Autodesk Inventor part; units mm, degrees
ref_plane "YZ Plane" through (0, 0, 0) normal (1, 0, 0) x (0, 1, 0)
ref_plane "XZ Plane" through (0, 0, 0) normal (0, 1, 0) x (-1, 0, 0)
ref_plane "XY Plane" through (0, 0, 0) normal (0, 0, 1) x (1, 0, 0)
sketch "Sketch1" plane through (0, 0, 0) normal (1, 0, 0) x (0, 1, 0)
  line L0 (9.8481, 428.814) -> (120.1519, 448.2635)
  line L1 (131.7365, 440.1519) -> (154.2135, 312.6787)
  line L2 (0, 78.3368) -> (0, 427.0775)
  line L3 (0, 417.0775) -> (0, 78.3368)
  line L4 (503.1119, 189.3047) -> (590.8645, 150.2346)
  line L5 (595.9326, 137.0318) -> (559.5861, 55.3964)
  line L6 (494.9423, 192.942) -> (494.9423, 192.942)
  line L7 (442.0149, 172.9748) -> (165.6696, 297.928)
  arc A0 (442.0149, 172.9748) -> (490.9347, 186.0198) centre (458.495, 209.4221) ccw
  arc A1 (154.2135, 312.6787) -> (165.6696, 297.928) centre (173.9096, 316.1516) ccw
  arc A2 (131.7365, 440.1519) -> (120.1519, 448.2635) centre (121.8884, 438.4154) ccw
  line L8 (9.8481, 428.814) -> (0, 417.0775)
  arc A3 (595.9326, 137.0318) -> (590.8645, 150.2346) centre (586.7972, 141.0991) ccw
  arc A4 (503.1119, 189.3047) -> (490.9347, 186.0198) centre (499.0446, 180.1692) ccw
  line L9 (9.651, 68.3429) -> (550.1017, 49.4699)
  arc A5 (550.1017, 49.4699) -> (559.5861, 55.3964) centre (550.4507, 59.4638) ccw
  arc A6 (0, 78.3368) -> (9.651, 68.3429) centre (10, 78.3368) ccw
  point P0 (0, 0)
  point P1 (0, 0)
  point P2 (130, 450)
  point P3 (156.0472, 302.2788)
  point P4 (0, 0)
  point P5 (534.922, 0)
  point P6 (600, 146.1672)
  point P7 (478.4622, 156.4947)
  point P8 (0, 427.0775)
  point P9 (537.6655, 6.1619)
  point P10 (0, 417.0775)
  dimension "d0" = 130
  dimension "d1" = 404.922
  dimension "d3" = 150
  dimension "d5" = 115
  dimension "d7" = 10
  dimension "d9" = 40
  dimension "d10" = 40
  dimension "d11" = 20
  dimension "d12" = 10
  dimension "d13" = 10
  dimension "d14" = 10
  dimension "d21" = 10
extrude "Extrusion1" add sketch "Sketch1" along normal blind 15
sketch "Sketch2" plane through (0, 0, 0) normal (-1, 0, 0) x (0, 0, 1)
  point P0 (0, 0)
sketch "Sketch3" plane through (0, 0, 0) normal (-1, 0, 0) x (0, 0, 1)
  line L0 (171.0338, 494.9772) -> (173.8576, 488.6347)
  line L1 (166.9664, 504.1126) -> (130.324, 487.7983)
  line L2 (130.324, 487.7983) -> (274.7158, 163.4898)
  line L3 (274.7158, 163.4898) -> (219.9031, 139.0856)
  line L4 (219.9031, 139.0856) -> (223.9704, 129.9501)
  line L5 (223.9704, 129.9501) -> (278.7831, 154.3544)
  line L6 (278.7831, 154.3544) -> (288.9516, 131.5158)
  line L7 (288.9516, 131.5158) -> (298.087, 135.5831)
  line L8 (298.087, 135.5831) -> (143.5268, 482.7303)
  line L9 (143.5268, 482.7303) -> (171.0338, 494.9772)
  line L10 (173.8576, 488.6347) -> (182.9931, 492.702)
  line L11 (182.9931, 492.702) -> (141.0991, 586.7972)
  line L12 (141.0991, 586.7972) -> (131.9637, 582.7298)
  line L13 (301.7603, 135.8301) -> (426.8309, 113.7768)
  line L14 (426.8309, 113.7768) -> (407.5559, 4.4631)
  line L15 (407.5559, 4.4631) -> (417.404, 2.7267)
  line L16 (417.404, 2.7267) -> (438.4154, 121.8884)
  line L17 (438.4154, 121.8884) -> (303.4968, 145.6782)
  line L18 (303.4968, 145.6782) -> (301.7603, 135.8301)
  line L19 (428.814, 9.8481) -> (417.0775, 0)
  line L20 (417.0775, 0) -> (78.3368, 0)
  line L21 (55.3964, 559.5861) -> (137.0318, 595.9326)
  arc A0 (150.2346, 590.8645) -> (137.0318, 595.9326) centre (141.0991, 586.7972) ccw
  line L22 (150.2346, 590.8645) -> (189.3047, 503.1119)
  arc A1 (186.0198, 490.9347) -> (189.3047, 503.1119) centre (180.1692, 499.0446) ccw
  arc A2 (186.0198, 490.9347) -> (172.9748, 442.0149) centre (209.4221, 458.495) ccw
  line L23 (172.9748, 442.0149) -> (297.928, 165.6696)
  arc A3 (297.928, 165.6696) -> (312.6787, 154.2135) centre (316.1516, 173.9096) ccw
  line L24 (312.6787, 154.2135) -> (440.1519, 131.7365)
  arc A4 (448.2635, 120.1519) -> (440.1519, 131.7365) centre (438.4154, 121.8884) ccw
  line L25 (448.2635, 120.1519) -> (428.814, 9.8481)
  line L26 (171.0338, 494.9772) -> (173.8576, 488.6347)
  line L27 (166.9664, 504.1126) -> (130.324, 487.7983)
  line L28 (130.324, 487.7983) -> (274.7158, 163.4898)
  line L29 (274.7158, 163.4898) -> (219.9031, 139.0856)
  line L30 (219.9031, 139.0856) -> (223.9704, 129.9501)
  line L31 (223.9704, 129.9501) -> (278.7831, 154.3544)
  line L32 (278.7831, 154.3544) -> (288.9516, 131.5158)
  line L33 (288.9516, 131.5158) -> (298.087, 135.5831)
  line L34 (298.087, 135.5831) -> (143.5268, 482.7303)
  line L35 (143.5268, 482.7303) -> (171.0338, 494.9772)
  line L36 (173.8576, 488.6347) -> (182.9931, 492.702)
  line L37 (182.9931, 492.702) -> (141.0991, 586.7972)
  line L38 (141.0991, 586.7972) -> (131.9637, 582.7298)
  line L39 (301.7603, 135.8301) -> (426.8309, 113.7768)
  line L40 (426.8309, 113.7768) -> (407.5559, 4.4631)
  line L41 (407.5559, 4.4631) -> (417.404, 2.7267)
  line L42 (417.404, 2.7267) -> (438.4154, 121.8884)
  line L43 (438.4154, 121.8884) -> (303.4968, 145.6782)
  line L44 (303.4968, 145.6782) -> (301.7603, 135.8301)
  line L45 (428.814, 9.8481) -> (417.0775, 0)
  line L46 (417.0775, 0) -> (78.3368, 0)
  line L47 (55.3964, 559.5861) -> (137.0318, 595.9326)
  arc A5 (150.2346, 590.8645) -> (137.0318, 595.9326) centre (141.0991, 586.7972) ccw
  line L48 (150.2346, 590.8645) -> (189.3047, 503.1119)
  arc A6 (186.0198, 490.9347) -> (189.3047, 503.1119) centre (180.1692, 499.0446) ccw
  arc A7 (186.0198, 490.9347) -> (172.9748, 442.0149) centre (209.4221, 458.495) ccw
  line L49 (172.9748, 442.0149) -> (297.928, 165.6696)
  arc A8 (297.928, 165.6696) -> (312.6787, 154.2135) centre (316.1516, 173.9096) ccw
  line L50 (312.6787, 154.2135) -> (440.1519, 131.7365)
  arc A9 (448.2635, 120.1519) -> (440.1519, 131.7365) centre (438.4154, 121.8884) ccw
  line L51 (448.2635, 120.1519) -> (428.814, 9.8481)
  line L52 (417.404, 2.7267) -> (438.4154, 121.8884)
  line L53 (58.3797, 539.0217) -> (136.0311, 573.5943)
  line L54 (54.3124, 548.1571) -> (141.0991, 586.7972)
  line L55 (136.0311, 573.5943) -> (131.9637, 582.7298)
  line L56 (141.0991, 586.7972) -> (182.9931, 492.702)
  line L57 (182.9931, 492.702) -> (173.8576, 488.6347)
  line L58 (166.9664, 504.1126) -> (136.0311, 573.5943)
  line L59 (166.9664, 504.1126) -> (130.324, 487.7983)
  line L60 (130.324, 487.7983) -> (274.7158, 163.4898)
  line L61 (274.7158, 163.4898) -> (219.9031, 139.0856)
  line L62 (219.9031, 139.0856) -> (223.9704, 129.9501)
  line L63 (223.9704, 129.9501) -> (278.7831, 154.3544)
  line L64 (278.7831, 154.3544) -> (288.9516, 131.5158)
  line L65 (288.9516, 131.5158) -> (298.087, 135.5831)
  line L66 (298.087, 135.5831) -> (143.5268, 482.7303)
  line L67 (143.5268, 482.7303) -> (171.0338, 494.9772)
  line L68 (171.0338, 494.9772) -> (173.8576, 488.6347)
  line L69 (303.4968, 145.6782) -> (301.7603, 135.8301)
  line L70 (301.7603, 135.8301) -> (426.8309, 113.7768)
  line L71 (426.8309, 113.7768) -> (407.5559, 4.4631)
  line L72 (407.5559, 4.4631) -> (417.404, 2.7267)
  line L73 (417.404, 2.7267) -> (438.4154, 121.8884)
  line L74 (438.4154, 121.8884) -> (303.4968, 145.6782)
  line L75 (131.9637, 582.7298) -> (54.3123, 548.1572)
  line L76 (54.3123, 548.1572) -> (58.3797, 539.0217)
  line L77 (58.3797, 539.0217) -> (136.0311, 573.5943)
  line L78 (136.0311, 573.5943) -> (166.9664, 504.1126)
  line L79 (68.3429, 9.651) -> (49.4699, 550.1017)
  arc A10 (55.3964, 559.5861) -> (49.4699, 550.1017) centre (59.4638, 550.4507) ccw
  arc A11 (68.3429, 9.651) -> (78.3368, 0) centre (78.3368, 10) ccw
  line L80 (131.9637, 582.7298) -> (54.3123, 548.1572)
  line L81 (54.3123, 548.1572) -> (58.3797, 539.0217)
  line L82 (58.3797, 539.0217) -> (136.0311, 573.5943)
  line L83 (136.0311, 573.5943) -> (166.9664, 504.1126)
  line L84 (68.3429, 9.651) -> (49.4699, 550.1017)
  arc A12 (55.3964, 559.5861) -> (49.4699, 550.1017) centre (59.4638, 550.4507) ccw
  arc A13 (68.3429, 9.651) -> (78.3368, 0) centre (78.3368, 10) ccw
  line L85 (54.3123, 548.1572) -> (58.3797, 539.0217)
  line L86 (73.2484, 352.9229) -> (142.3938, 197.6203)
  line L87 (142.3938, 197.6203) -> (156.0969, 203.7213)
  line L88 (156.0969, 203.7213) -> (86.9516, 359.024)
  line L89 (86.9516, 359.024) -> (73.2484, 352.9229)
  line L90 (73.2484, 352.9229) -> (142.3938, 197.6203)
  line L91 (142.3938, 197.6203) -> (156.0969, 203.7213)
  line L92 (156.0969, 203.7213) -> (86.9516, 359.024)
  line L93 (86.9516, 359.024) -> (73.2484, 352.9229)
  line L94 (86.9516, 359.024) -> (156.0969, 203.7213)
  line L95 (142.3938, 197.6203) -> (156.0969, 203.7213)
  line L96 (142.3938, 197.6203) -> (73.2484, 352.9229)
  line L97 (73.2484, 352.9229) -> (86.9516, 359.024)
  point P0 (0, 0)
  point P1 (131.9642, 582.73)
extrude "Extrusion2" cut sketch "Sketch3" against normal blind 7 contours L9 L8 L7 L6 L5 L4 L3 L2 L1 L58 L55 L12 L11 L10 L0 | L55 L53 L76 L54 | L18 L17 L16 L15 L14 L13 | L89 L88 L87 L86
properties part number "Arcade_Right"
Read the model definition and answer for the solid it produces. Units are mm, in the model's axes. A direction names the side the tool comes from. Coordinates: 2 decimals unless noted, no trailing zeros. Order: outer loops, then holes, each group sorted by start corner. A loop starts at its lowest first (then second) coordinate and runs counter-clockwise, first axis right, second up. Notation, with made-up numbers: M 5.25,26 L 56.25,26 A7 cw 56.25,31 Z; hole C -10,11 d9. An arc over 180 degrees is marked long. Put each result on its own line as item: value. Start each with the question number.
Item 1: Given pin 1 Ø1.5 at (x, z) = (12.5, 323.5) entering from +Y; pin 2 Ø6 at (x, y) = (5, 351) entering from -Z; pin 3 Ø1 at (y, z) = (205, 103) entering from -X; pin 4 Ø6 at (x, y) = (8.5, 67) entering from -Z, each flat-ended and moving along its own axis, determine where each tip first touches the part or whether it passes through.
Item 2: Section C-C, the plane x = 11 is taken. Determine the outline of the cut face in (y, z) (1 decimal).
Item 3: For faces 1 (the face through (7.4, 596.09, 144.79)), 2 (the face through (3.5, 280.3, 122)), determine the directions among +Z, -Z, +X, -X, +Y, -Y from which every point of the face is accessible in a straight line to the end or side of a thin tool.
Item 4: Section B-B, the plane z = 373 is taken. Determine the outline of the cut face in (x, y).
Item 5: Section A-A, the plane y = 64.5 is taken. Determine the outline of the cut face in (x, z), plus the area to 3 significant figures.
Item 6: Section D-D, the plane z = 262.5 is taken. Determine the outline of the cut face in (x, y), plus the area to 3 significant figures.
Item 7: The mould has two halves that part along Z. Classify faces 3 (the face through (7, 0, 245)), 4 (the face through (3.5, 306.7, 221.9)), 5 (the face through (7.395, 142.818, 377.308)), 6 (the face through (3.451, 124.958, 363.42)): +Z half, -Z half, draft (parallel to the pull), parting line (faces both ways), or undercut.
Item 8: Consider probe 1 along Y at (x, z) = (4.25, 75.5); probe 2 along Y at (x, z) = (5.5, 154.5); probe 3 along Y at (x, z) = (3, 269). Determine where each line is inside the solid, lowest interval first. Write a range as [from, to].
Computed:
1. pin 1: stops at y = 152.44
1. pin 2: stops at z = 56.32
1. pin 3: stops at x = 0
1. pin 4: stops at z = 66.24
2. outline: M 0,78.3 A10 ccw 9.7,68.3 L 550.1,49.5 A10 ccw 559.6,55.4 L 595.9,137 A10 ccw 590.9,150.2 L 503.1,189.3 A10 ccw 490.9,186 A40 cw 442,173 L 165.7,297.9 A20 cw 154.2,312.7 L 131.7,440.2 A10 ccw 120.2,448.3 L 9.8,428.8 L 0,417.1 Z
3. face 1: +X, -X, +Y
3. face 2: -X
4. outline: M 0,0 L 15,0 L 15,143.58 L 0,143.58 L 0,133.42 L 7,133.42 L 7,123.27 L 0,123.27 Z
5. outline: M 0,66.43 L 15,66.43 L 15,438.45 L 0,438.45 L 0,428.3 L 7,428.3 L 7,418.14 L 0,418.14 Z
5. area: 5,510 mm2
6. outline: M 0,0 L 15,0 L 15,244.02 L 0,244.02 L 0,215.51 L 7,215.51 L 7,190.93 L 0,190.93 L 0,158.05 L 7,158.05 L 7,147.1 L 0,147.1 Z
6. area: 3,410 mm2
7. face 3: draft
7. face 4: undercut
7. face 5: +Z half
7. face 6: undercut
8. probe 1: y = [0.41, 347.87], [353.93, 546.64], [557.59, 568.54]
8. probe 2: y = [0, 203.01], [207.31, 433.5], [458.08, 487.62], [498.56, 532.11], [556.7, 581.28]
8. probe 3: y = [0, 150], [160.94, 176.33], [200.91, 229.65]
